```python
from build123d import *

# Parameters (mm, degrees)
SKETCH1_R                = 10
BOSS_EXTRUDE1_DEPTH      = 7.25
BOSS_EXTRUDE1_DEPTH_BACK = 7.25
SKETCH2_W                = 45
SKETCH2_H                = 45
BOSS_EXTRUDE2_DEPTH      = 60
SKETCH3_R                = 10
BOSS_EXTRUDE3_DEPTH      = 15


with BuildPart() as part:
    # Sketch1 → Boss-Extrude1 (new body, two sides)
    with BuildSketch(Plane.XY) as boss_extrude1_sk:
        with BuildLine():
            Line((0, 22.5), (0, -22.5))
            Line((0, -22.5), (-35, -22.5))
            ThreePointArc((-35, -22.5), (-57.5, 0), (-35, 22.5))
            Line((-35, 22.5), (0, 22.5))
        make_face()
        with Locations((-35, 0)):
            Circle(SKETCH1_R, mode=Mode.SUBTRACT)
    extrude(amount=BOSS_EXTRUDE1_DEPTH)
    extrude(boss_extrude1_sk.sketch, amount=-BOSS_EXTRUDE1_DEPTH_BACK)

    # Sketch2 → Boss-Extrude2 (add)
    with BuildSketch(Plane(origin=(0, 0, 0), x_dir=(0, 0, -1), z_dir=(1, 0, 0))):
        Rectangle(SKETCH2_W, SKETCH2_H)
    extrude(amount=BOSS_EXTRUDE2_DEPTH)

    # Sketch3 → Boss-Extrude3 (add)
    with BuildSketch(Plane.XY.offset(7.5)):
        with BuildLine():
            Line((60, 22.5), (60, -22.5))
            Line((60, -22.5), (95, -22.5))
            ThreePointArc((95, -22.5), (117.5, 0), (95, 22.5))
            Line((95, 22.5), (60, 22.5))
        make_face()
        with Locations((95, 0)):
            Circle(SKETCH3_R, mode=Mode.SUBTRACT)
    boss_extrude3 = extrude(amount=BOSS_EXTRUDE3_DEPTH)

    # Mirror1: Boss-Extrude3 across plane
    add(boss_extrude3.mirror(Plane.XY))


solid = part.part
```
For this review, take the finished solid that the model builds, in its own axes (mm). A direction names the side the tool comes from. Round coordinates to 2 decimals unless told otherwise and drop trailing zeros. Write each loop counter-clockwise with the first axis right and the second up, starting at its lowest first coordinate (ties: lowest second). Pieces come first, ordered by that corner, then holes. Notation, with made-up numbers: (41.25, -6.75) - (82.25, -6.75) arc R21 ccw to (82.25, 2.25) - close; hole circle Ø4 at (68, 77). An arc over 180 degrees is marked (long way). Answer as a JSON object with one key per item and string values.
1. We need section D-D on x = 93. Give the boundary of the cut face in (y, z), then the cut area to 3 significant figures.
Response values:
{"outline": "(-22.5, -22.5) - (-9.8, -22.5) - (-9.8, -7.5) - (-22.5, -7.5) - close; (-22.5, 7.5) - (-9.8, 7.5) - (-9.8, 22.5) - (-22.5, 22.5) - close; (9.8, -22.5) - (22.5, -22.5) - (22.5, -7.5) - (9.8, -7.5) - close; (9.8, 7.5) - (22.5, 7.5) - (22.5, 22.5) - (9.8, 22.5) - close", "area": "762 mm2"}
2. For pin 1 Ø6 at (y, z) = (-13.5, 11.5) entering from +X; pin 2 Ø7.5 at (y, z) = (-2.5, 2.5) entering from +X; pin 3 Ø5 at (y, z) = (12, -0.5) entering from -X, all flat-tipped, find the tip position at first contact; note any pin that passes through.
Response values:
{"pin 1": "stops at x = 114.9", "pin 2": "stops at x = 60", "pin 3": "stops at x = -55.4"}
3. We need section A-A on y = 0. Give the boundary of the cut face in (x, z).
Response values:
{"outline": "(-57.5, -7.25) - (-45, -7.25) - (-45, 7.25) - (-57.5, 7.25) - close; (-25, -7.25) - (0, -7.25) - (0, -22.5) - (85, -22.5) - (85, -7.5) - (60, -7.5) - (60, 7.5) - (85, 7.5) - (85, 22.5) - (0, 22.5) - (0, 7.25) - (-25, 7.25) - close; (105, -22.5) - (117.5, -22.5) - (117.5, -7.5) - (105, -7.5) - close; (105, 7.5) - (117.5, 7.5) - (117.5, 22.5) - (105, 22.5) - close"}
4. We need section C-C on y = -18. Give the boundary of the cut face in (x, z), then the cut area to 3 significant figures.
Response values:
{"outline": "(-48.5, -7.25) - (0, -7.25) - (0, -22.5) - (108.5, -22.5) - (108.5, -7.5) - (60, -7.5) - (60, 7.5) - (108.5, 7.5) - (108.5, 22.5) - (0, 22.5) - (0, 7.25) - (-48.5, 7.25) - close", "area": "4,860 mm2"}
5. We need section B-B on z = 9. Give the boundary of the cut face in (x, y).
Response values:
{"outline": "(0, -22.5) - (95, -22.5) arc R22.5 ccw to (95, 22.5) - (0, 22.5) - close; hole circle Ø20 at (95, 0)"}
6. Tool access review of faces 1 (the face through (-45, 0, 0)), 2 (the face through (-22, 0, -7.25)), 3 (the face through (58, 0, -22.5)), 4 (the face through (82, 0, -7.5)), 5 (the face through (0, 0, 15)): name each direction out of +Z, -Z, +X, -X, +Y, -Y from which nothing blocks a thin tool from reaching the whole face with its end or side.
Response values:
{"face 1": "+Z, -Z", "face 2": "-Z, -X, +Y, -Y", "face 3": "-Z, +X, -X, +Y, -Y", "face 4": "+X, +Y, -Y", "face 5": "+Z, -X, +Y, -Y"}
7. To check wall thickness, follow line 1 along Y through (x, z) = (-35, 1.25); line 2 along Z through (x, y) = (109, -15); line 3 along X through (y, z) = (-5.5, -3). State the ranges of each line that lie inside material, in increasing order.
Response values:
{"line 1": "y = -22.5 to -10, 10 to 22.5", "line 2": "z = -22.5 to -7.5, 7.5 to 22.5", "line 3": "x = -56.82 to -43.35, -26.65 to 60"}
8. Draft analysis for pull direction X (two halves, no side actions). For faces 6 (the face through (85, 0, 15)), 7 (the face through (60, 0, 0)), 8 (the face through (58, 0, 22.5)), state which applies: +X half, -X half, draft (parallel to the pull), parting line (faces both ways), or undercut.
Response values:
{"face 6": "undercut", "face 7": "+X half", "face 8": "draft"}
